Part model, mm, in its own coordinate system. A direction names the side the tool comes from. Round coordinates to 2 decimals unless told otherwise and drop trailing zeros. Loops run counter-clockwise (first coordinate to the right, second up) from the corner with the lowest first, then second, coordinate; pieces in that order, holes last. Notation, with made-up numbers: (80, 25) - (129, 25) arc R17 ccw to (129, 43) - close; hole circle Ø4 at (1.25, -17.5). An arc over 180 degrees is marked (long way). Put each result on its own line as item: value.
from build123d import *


with BuildPart() as part:
    # Sketch1 → Revolve1 (revolve)
    with BuildSketch(Plane(origin=(0, 0, 0), x_dir=(0, 0, -1), z_dir=(1, 0, 0)), mode=Mode.PRIVATE) as revolve1_sk:
        with BuildLine():
            Line((2, 32.625), (3, 32.625))
            Line((3, 32.625), (3, 32.675))
            Line((3, 32.675), (36.3, 32.675))
            Line((36.3, 32.675), (36.8, 32.175))
            Line((36.8, 32.175), (36.8, 29.5))
            Line((36.8, 29.5), (32.12346282, 21.4))
            ThreePointArc((32.12346282, 21.4), (31.391412012, 20.667949192), (30.391412012, 20.4))
            Line((30.391412012, 20.4), (17.599342077, 20.4))
            ThreePointArc((17.599342077, 20.4), (15.50769201, 20.858524469), (13.799671038, 22.15))
            ThreePointArc((13.799671038, 22.15), (12.091650066, 23.441475531), (10, 23.9))
            Line((10, 23.9), (1, 23.9))
            ThreePointArc((1, 23.9), (0.292893219, 24.192893219), (0, 24.9))
            Line((0, 24.9), (0, 30.625))
            Line((0, 30.625), (2, 32.625))
        make_face()
    revolve(revolve1_sk.sketch.rotate(Axis((0, 0, 0), (0, 0, -1)), 90), axis=Axis((0, 0, 0), (0, 0, -1)))


solid = part.part
1. Pin check, flat tips, straight feed: P1, Ø2, axis at x = 14, z = -9, coming from the -Y side; P2, Ø5, axis at x = -15, z = -31, coming from the -Y side; P3, Ø12, axis at x = 13.5, y = -3.5, coming from the -Z side; P4, Ø3, axis at x = 5.5, z = -32.5, coming from the +Y side. Stop position of each tip, or through.
A:
P1: stops at y = -29.98
P2: stops at y = -30.19
P3: passes through
P4: stops at y = 32.43
2. Band-saw the part on A-A (z = -21.5). List the corners of the cut face in (x, y) (3 decimals), plus the area to 3 significant figures.
A:
outline: circle Ø65.35 at (0, 0); hole circle Ø40.8 at (0, 0)
area: 2,050 mm²
3. Probe line 1 along Y through (x, z) = (0, -23) (3 decimals); line 2 along Y through (x, z) = (0, -3) (3 decimals); line 3 along X through (y, z) = (-15, -8.5). List the from-to ranges inside material, lowest first. Write a range as [from, to].
A:
line 1: y = [-32.675, -20.4], [20.4, 32.675]
line 2: y = [-32.625, -23.9], [23.9, 32.625]
line 3: x = [-29.03, -18.61], [18.61, 29.03]
4. Two-plate mould, pull along X, no slides. Class faces 1 (the conical face through (-17.29, 13.26, -32.35)), 2 (the flat face through (14.1, 26.1, -36.8)), 3 (the conical face through (14.189, 27.281, -0.125)): pulls with the +X half, pulls with the -X half, needs draft (parallel to the pull), parting line crosses it, or undercut.
A:
face 1: undercut
face 2: needs draft
face 3: parting line crosses it
5. Tool access for faces 4 (the cylindrical face through (19.458, -6.128, -23.906)), 5 (the cylindrical face through (12.85, -20.15, -5.44)): list every direction of +Z, -Z, +X, -X, +Y, -Y with a clear straight run to the whole face (end or side of a thin tool).
A:
face 4: +Z, -Z
face 5: +Z
6. Band-saw the part on B-B (z = -5). List the corners of the cut face in (x, y) (3 decimals).
A:
outline: circle Ø65.35 at (0, 0); hole circle Ø47.8 at (0, 0)
